Input: part model. Units: mm. Frame: model coordinates. A direction names the side the tool comes from. Round coordinates to 2 decimals unless told otherwise and drop trailing zeros. Loops run counter-clockwise (first coordinate to the right, second up) from the corner with the lowest first, then second, coordinate; pieces in that order, holes last. Notation, with made-up numbers: (29, 68.25) - (74, 68.25) arc R21 cw to (74, 99.25) - close; hole circle Ø9 at (-28.5, -9.5). An arc over 180 degrees is marked (long way). Write each question's results on one line, items separated by ' | '.
from build123d import *

# Parameters (mm, degrees)
SKETCH002_R  = 1.5
PAD003_DEPTH = 5
PAD002_DEPTH = 2
SKETCH_W     = 45
SKETCH_H     = 20
SKETCH_R     = 1.8
PAD_DEPTH    = 3
PAD001_DEPTH = 20


with BuildPart() as mount:
    # Sketch002 → Pad003 (new body)
    with BuildSketch(Plane.XZ.offset(10)):
        with Locations((0, 6)):
            Circle(SKETCH002_R)
        with BuildLine():
            ThreePointArc((1.5, 21), (0, 22.5), (-1.5, 21))
            Line((-1.5, 21), (-1.5, 19))
            ThreePointArc((-1.5, 19), (0, 17.5), (1.5, 19))
            Line((1.5, 21), (1.5, 19))
        make_face()
    extrude(amount=-PAD003_DEPTH)


with BuildPart() as cutblock:
    # Sketch003 → Pad002 (new body)
    with BuildSketch(Plane(origin=(0, -5, 0), x_dir=(-1, 0, 0), z_dir=(0, 1, 0))):
        Polygon((-1.5, 3.401924), (1.5, 3.401924), (3, 6), (1.5, 8.598076), (-1.5, 8.598076), (-3, 6), align=None)
        Polygon((2.598075, 16.499999), (2.598075, 23), (0, 24.499999), (-2.598075, 23), (-2.598075, 16.499999), (0, 15), align=None)
    extrude(amount=-PAD002_DEPTH)

    # Fusion001: union Mount
    add(mount.part)


with BuildPart() as base:
    # Sketch → Pad (new body)
    with BuildSketch(Plane.XY):
        Rectangle(SKETCH_W, SKETCH_H)
        with Locations((-6, 5)):
            Circle(SKETCH_R, mode=Mode.SUBTRACT)
        with Locations((6, 5)):
            Circle(SKETCH_R, mode=Mode.SUBTRACT)
        with Locations((-18.5, -5)):
            Circle(SKETCH_R, mode=Mode.SUBTRACT)
        with Locations((18.5, -5)):
            Circle(SKETCH_R, mode=Mode.SUBTRACT)
    extrude(amount=PAD_DEPTH)


with BuildPart() as final:
    # Sketch001 → Pad001 (new body)
    with BuildSketch(Plane.XY.offset(3)):
        Polygon((-12, 0), (-15.90274, 0), (-15.90274, -10), (15.90274, -10), (15.90274, 0), (12, 0), (12, -5), (-12, -5), align=None)
    extrude(amount=PAD001_DEPTH)

    # Fusion: union Base
    add(base.part)

    # Cut: cut CutBlock
    add(cutblock.part, mode=Mode.SUBTRACT)


solid = final.part
1. Contact query for flat-ended pins moving along their axis: pin 1 (1.6 mm diameter, centred on y = -6, z = 19, fed in from -X); pin 2 (1.6 mm diameter, centred on y = -6, z = 21, fed in from +X); pin 3 (3 mm diameter, centred on x = 18.5, y = -5, fed in from -Z); pin 4 (6 mm diameter, centred on x = 4.5, z = 11, fed in from +Y). Output: stop coordinate, or through.
Answer:
pin 1: x = -15.9 | pin 2: x = 15.9 | pin 3: through | pin 4: y = -5
2. Section query A-A, the plane x = -18.5. Output: boundary loops of the cut face in (y, z), plus the area to 3 significant figures.
Answer:
outline: (-10, 0) - (-6.8, 0) - (-6.8, 3) - (-10, 3) - close; (-3.2, 0) - (10, 0) - (10, 3) - (-3.2, 3) - close | area: 49.2 mm^2
3. Section query B-B, the plane y = -6. Output: boundary loops of the cut face in (x, z).
Answer:
outline: (-22.5, 0) - (-20, 0) - (-20, 3) - (-22.5, 3) - close; (-17, 0) - (17, 0) - (17, 3) - (15.9, 3) - (15.9, 23) - (2.6, 23) - (2.6, 16.5) - (0, 15) - (-2.6, 16.5) - (-2.6, 23) - (-15.9, 23) - (-15.9, 3) - (-17, 3) - close; (20, 0) - (22.5, 0) - (22.5, 3) - (20, 3) - close; hole (-3, 6) - (-1.5, 3.4) - (1.5, 3.4) - (3, 6) - (1.5, 8.6) - (-1.5, 8.6) - close
4. Section query C-C, the plane z = 6.5. Output: boundary loops of the cut face in (x, y), plus the area to 3 significant figures.
Answer:
outline: (-15.9, -10) - (-1.41, -10) - (-1.41, -7) - (-2.71, -7) - (-2.71, -5) - (-12, -5) - (-12, 0) - (-15.9, 0) - close; (1.41, -10) - (15.9, -10) - (15.9, 0) - (12, 0) - (12, -5) - (2.71, -5) - (2.71, -7) - (1.41, -7) - close | area: 179 mm^2
5. Mould query, pull axis Z, two halves, no side actions, for faces 5 (the flat face through (2.598, -6, 20)), 6 (the flat face through (2.26, -5.99, 4.72)), 7 (the flat face through (-0.2, -7.2, 23)). Classes: pulls with the +Z half, pulls with the -Z half, needs draft (parallel to the pull), parting line crosses it, or undercut.
Answer:
face 5: needs draft | face 6: undercut | face 7: pulls with the +Z half
6. Set-up query: faces 1 (the flat face through (2.24, -5.99, 7.32)), 2 (the cylindrical face through (-18.734, -3.215, 1.479)), 3 (the flat face through (-1.5, -9, 20)), 4 (the flat face through (-12, -3, 13)). Return all of +Z, -Z, +X, -X, +Y, -Y with unobstructed straight access to the full face (end or side cutting, diameter ignored); none if empty.
Answer:
face 1: +Y | face 2: +Z, -Z | face 3: +Y, -Y | face 4: +Z, +Y
7. Line query: line 1 (Z direction, x = 0, y = -8.05); line 2 (X direction, y = -0.75, z = 5.5); line 3 (Y direction, x = 6, z = 0.9). Output: solid intervals per line, ascending. Write a range as [from, to].
Answer:
line 1: [0, 4.5], [7.5, 17.5], [22.5, 23] | line 2: [-15.9, -12], [12, 15.9] | line 3: [-10, 3.2], [6.8, 10]
8. Section query D-D, the plane z = 12.5. Output: boundary loops of the cut face in (x, y).
Answer:
outline: (-15.9, -10) - (15.9, -10) - (15.9, 0) - (12, 0) - (12, -5) - (-12, -5) - (-12, 0) - (-15.9, 0) - close
